from build123d import *

# Parameters (mm, degrees)
F1_DEPTH = 10
F2_T     = -1


with BuildPart() as f1:
    # F0 (on Top) → F1 (new body)
    with BuildSketch(Plane.XY):
        Polygon((-14.713825658, 44.3513132632), (-44.7570756078, 44.3513132632), (-44.3209633231, -44.5757396519), (-14.713825658, -44.5757396519), (-14.713825658, -14.638537541), (14.726145193, -14.638537541), (14.726145193, -44.034704566), (44.1661179066, -44.034704566), (44.1661179066, -14.3647896479), (58.8016323745, 0), (44.1661179066, 14.9113414809), (44.1661179066, 44.3513132632), (14.726145193, 44.3513132632), (14.726145193, 14.9113414809), (-14.713825658, 14.9113414809), align=None)
    extrude(amount=F1_DEPTH)

    # F2
    f2_openings = [f1.faces().sort_by_distance(p)[0] for p in [
        (1.349814, 0.088253, 0),
    ]]
    offset(amount=F2_T, openings=f2_openings, kind=Kind.INTERSECTION)


solid = f1.part
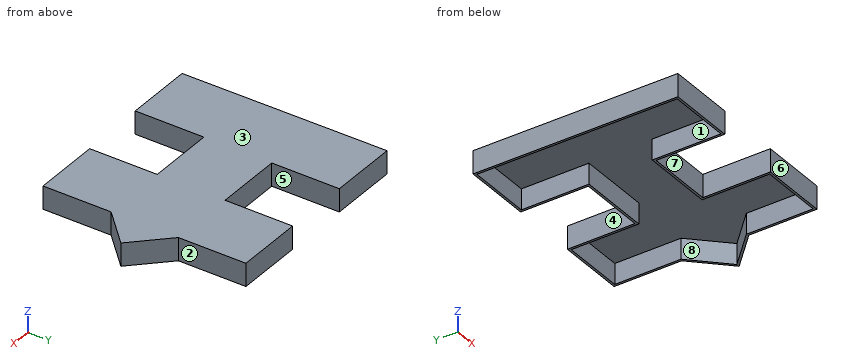
Work out the finished part from the listing and answer in its coordinate system (mm). Face numbers are marked on the shaded views. A direction names the side the tool comes from. Give positions to 0.01 mm unless a question says otherwise; leave off trailing zeros. Loops run counter-clockwise (first coordinate to the right, second up) from the corner with the lowest first, then second, coordinate; pieces in that order, holes last. Notation, with made-up numbers: (-32.5, -29.5) -> (-7.5, -29.5) arc R21 cw to (-7.5, 8.5) -> close; hole circle Ø6 at (-25, 61.5). An arc over 180 degrees is marked (long way). Use a Markdown table: item, result. Add a question column.
1) For a pull along X with two mould halves and no side action, classify the marked faces 1, 2, 3 and 4 as +X half, -X half, draft (parallel to the pull), parting line (faces both ways), or undercut.
2) Consider line 1 along X through (y, z) = (-39, 6.75); line 2 along X through (y, z) = (39.5, 2.75); line 3 along Y through (x, z) = (-21, 7). Determine where each line is inside the solid, lowest interval first.
3) The part is cut by section D-D, the plane y = 6.5. Determine the outline of the cut face in (x, z), plus the area to 3 significant figures.
4) Each of these flat-tipped pins is pushed along its axis until it touches: P1, Ø1.5, axis at y = -10.5, z = 5, coming from the +X side; P2, Ø3, axis at y = 2, z = 7, coming from the -X side; P3, Ø4.5, axis at y = -34.5, z = 4, coming from the -X side. Where does it stop, or does it pass through?
5) The part is cut by section C-C, the plane x = -35.5. Determine the outline of the cut face in (y, z), plus the area to 3 significant figures.
6) Which of the six approach directions +Z, -Z, +X, -X, +Y, -Y give full straight-line access (tool end or side, diameter ignored) to the marked faces 5, 6, 7 and 8?
7) The part is cut by section B-B, the plane y = 35. Determine the outline of the cut face in (x, z).
Reported:
| question | item | result |
|---|---|---|
| 1 | face 1 | undercut |
| 1 | face 2 | +X half |
| 1 | face 3 | draft |
| 1 | face 4 | undercut |
| 2 | line 1 | x = -44.35 to -43.35, -15.71 to -14.71, 14.73 to 15.73, 43.17 to 44.17 |
| 2 | line 2 | x = -44.73 to -43.73, -15.71 to -14.71, 14.73 to 15.73, 43.17 to 44.17 |
| 2 | line 3 | y = -44.58 to -43.58, 43.35 to 44.35 |
| 3 | outline | (-44.57, 0) -> (-43.57, 0) -> (-43.57, 9) -> (51.02, 9) -> (51.02, 0) -> (52.42, 0) -> (52.42, 10) -> (-44.57, 10) -> close |
| 3 | area | 119 mm^2 |
| 4 | P1 | stops at x = 48.87 |
| 4 | P2 | stops at x = -44.56 |
| 4 | P3 | stops at x = -44.38 |
| 5 | outline | (-44.58, 0) -> (-43.58, 0) -> (-43.58, 9) -> (43.35, 9) -> (43.35, 0) -> (44.35, 0) -> (44.35, 10) -> (-44.58, 10) -> close |
| 5 | area | 107 mm^2 |
| 6 | face 5 | +Z, -Z, +Y |
| 6 | face 6 | +Z, -Z, +X, -Y |
| 6 | face 7 | +Z, -Z, -Y |
| 6 | face 8 | -Z |
| 7 | outline | (-44.71, 0) -> (-43.71, 0) -> (-43.71, 9) -> (-15.71, 9) -> (-15.71, 0) -> (-14.71, 0) -> (-14.71, 10) -> (-44.71, 10) -> close; (14.73, 0) -> (15.73, 0) -> (15.73, 9) -> (43.17, 9) -> (43.17, 0) -> (44.17, 0) -> (44.17, 10) -> (14.73, 10) -> close |
